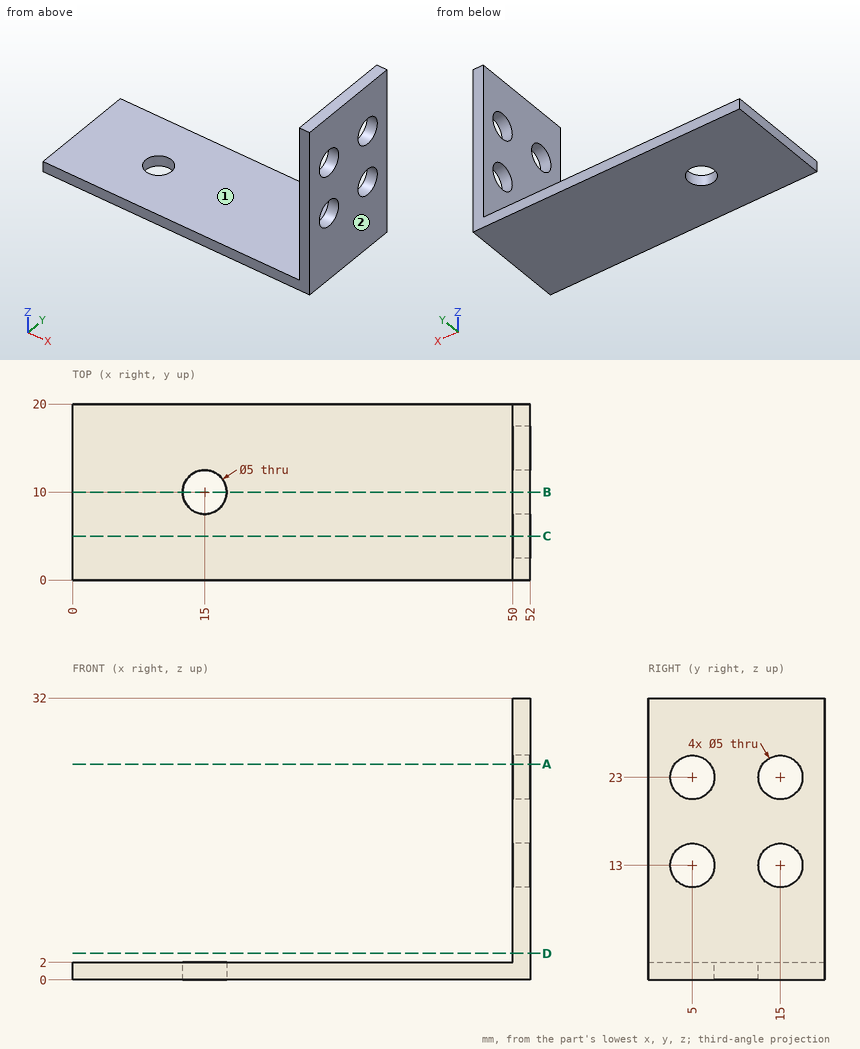
For this review, use the dimensioned drawing (mm, ordinates from the lowest corner) and the shaded views. A direction names the side the tool comes from. Coordinates: 2 decimals unless noted, no trailing zeros. Loops run counter-clockwise (first coordinate to the right, second up) from the corner with the lowest first, then second, coordinate; pieces in that order, holes last. Notation, with made-up numbers: (31.25, 78.5) - (78.25, 78.5) arc R18 cw to (78.25, 105.5) - close; hole circle Ø2 at (61.25, 42). An arc over 180 degrees is marked (long way). Use one line per item in the form item = value. Start each with the question number.
1) For the marked faces 1 and 2, list the 3-axis set-ups (+Z, -Z, +X, -X, +Y, -Y) from which the entire face can be reached by the end or side of a thin tool; tool diameter is ignored.
2) To check wall thickness, follow probe 1 along Z at (x, y) = (51.3, 15); probe 2 along Y at (x, z) = (51.1, 13); probe 3 along Y at (x, z) = (50.5, 14.5). State the ranges of each line that lie inside material, in increasing order. Write a range as from..to.
3) For pin 1 (1 mm diameter, centred on x = 28.5, y = 15.5, fed in from -Z); pin 2 (3 mm diameter, centred on y = 3.5, z = 8, fed in from -X); pin 3 (8 mm diameter, centred on x = 17, y = 5.5, fed in from +Z), all flat-tipped, find the tip position at first contact; note any pin that passes through.
4) Take a section at D-D (z = 3). State the section outline as (x, y) points, plus the area to 3 significant figures.
5) Take a section at C-C (y = 5). State the section outline as (x, z) points, plus the area to 3 significant figures.
6) Take a section at A-A (z = 24.5). State the section outline as (x, y) points.
7) Take a section at B-B (y = 10). State the section outline as (x, z) points.
From the geometry:
q1.face_1 = +Z, -X, +Y, -Y
q1.face_2 = +Z, -Z, +X, +Y, -Y
q2.probe_1 = 0..10.5, 15.5..20.5, 25.5..32
q2.probe_2 = 0..2.5, 7.5..12.5, 17.5..20
q2.probe_3 = 0..3, 7..13, 17..20
q3.pin_1 = 0
q3.pin_2 = 50
q3.pin_3 = 2
q4.outline = (50, 0) - (52, 0) - (52, 20) - (50, 20) - close
q4.area = 40.0 mm2
q5.outline = (0, 0) - (52, 0) - (52, 10.5) - (50, 10.5) - (50, 2) - (0, 2) - close; (50, 15.5) - (52, 15.5) - (52, 20.5) - (50, 20.5) - close; (50, 25.5) - (52, 25.5) - (52, 32) - (50, 32) - close
q5.area = 144 mm2
q6.outline = (50, 0) - (52, 0) - (52, 3) - (50, 3) - close; (50, 7) - (52, 7) - (52, 13) - (50, 13) - close; (50, 17) - (52, 17) - (52, 20) - (50, 20) - close
q7.outline = (0, 0) - (12.5, 0) - (12.5, 2) - (0, 2) - close; (17.5, 0) - (52, 0) - (52, 32) - (50, 32) - (50, 2) - (17.5, 2) - close
